```python
from build123d import *

# Parameters (mm, degrees)
CUT_EXTRUDE1_START        = -45.212
CUT_EXTRUDE1_DEPTH        = 3.302
CUT_EXTRUDE1_DEPTH_BACK   = 1.5875
SKETCH4_W                 = 30.1625
SKETCH4_H                 = 23.495
BOSS_EXTRUDE1_DEPTH       = 3.175
SKETCH5_R                 = 1.524
CUT_EXTRUDE2_DEPTH        = 8.96925
F_1_0MM_DOWEL_HOLE1_D     = 1
F_1_0MM_DOWEL_HOLE1_DEPTH = 3.175


with BuildPart() as part:
    # Sketch2 → Revolve1 (revolve)
    with BuildSketch(Plane.XY):
        Polygon((45.24375, -12.7), (50.00625, -12.7), (50.00625, 9.525), (54.76875, 9.525), (54.76875, 12.7), (50.00625, 12.7), (45.24375, 12.7), align=None)
    revolve(axis=Axis((0, 12.7, 0), (0, -1, 0)))

    # Sketch3 → Cut-Extrude1 (cut, two sides)
    with BuildSketch(Plane.XY.offset(CUT_EXTRUDE1_START)) as cut_extrude1_sk:
        with BuildLine():
            Line((-15.08125, -12.7), (15.08125, -12.7))
            Line((15.08125, -12.7), (15.08125, -5.55625))
            ThreePointArc((15.08125, -5.55625), (0, 9.525), (-15.08125, -5.55625))
            Line((-15.08125, -5.55625), (-15.08125, -12.7))
        make_face()
    extrude(amount=CUT_EXTRUDE1_DEPTH, mode=Mode.SUBTRACT)
    extrude(cut_extrude1_sk.sketch, amount=-CUT_EXTRUDE1_DEPTH_BACK, mode=Mode.SUBTRACT)

    # Sketch4 → Boss-Extrude1 (add)
    with BuildSketch(Plane.XY.offset(-46.7995)):
        with BuildLine():
            ThreePointArc((15.08125, -5.55625), (0, 9.525), (-15.08125, -5.55625))
            Line((-15.08125, -5.55625), (-15.08125, -12.7))
            Line((-15.08125, -12.7), (15.08125, -12.7))
            Line((15.08125, -12.7), (15.08125, -5.55625))
        make_face()
        with Locations((0, -24.4475)):
            Rectangle(SKETCH4_W, SKETCH4_H)
    extrude(amount=-BOSS_EXTRUDE1_DEPTH)

    # Sketch5 → Cut-Extrude2 (cut, through all)
    with BuildSketch(Plane.XY.offset(-46.7995)):
        with Locations((0, -19.0881)):
            Circle(SKETCH5_R)
        with Locations((0, -9.3091)):
            Circle(SKETCH5_R)
        with BuildLine():
            Line((-3.175, -36.195), (-3.175, -28.9687))
            ThreePointArc((-3.175, -28.9687), (0, -25.7937), (3.175, -28.9687))
            Line((3.175, -28.9687), (3.175, -36.195))
            Line((3.175, -36.195), (-3.175, -36.195))
        make_face()
    extrude(amount=-CUT_EXTRUDE2_DEPTH, mode=Mode.SUBTRACT)

    # Ø1.0mm Dowel Hole1
    with Locations(Plane(origin=(0, 9.525, 0), x_dir=(-1, 0, 0), z_dir=(0, -1, 0))):
        with Locations((-35.279486504, -38.727354522), (-37.043556499, 37.043556499), (37.043556499, 37.043556499), (37.043556499, -37.043556499)):
            Hole(F_1_0MM_DOWEL_HOLE1_D / 2, depth=F_1_0MM_DOWEL_HOLE1_DEPTH)


solid = part.part
```
The model under review builds one solid part; all positions refer to its coordinate system, in mm. A direction names the side the tool comes from. Round coordinates to 2 decimals unless told otherwise and drop trailing zeros. Order: outer loops, then holes, each group sorted by start corner. A loop starts at its lowest first (then second) coordinate and runs counter-clockwise, first axis right, second up.
Item 1: Draft analysis for pull direction X (two halves, no side actions). For faces 5 (the flat face through (9, -36.195, -48)), 6 (the cylindrical face through (-7.13, 11.135, 54.303)), 7 (the flat face through (15.081, -9, -45)), 8 (the cylindrical face through (0.33, 9.52, -45.68)), state which applies: released by +X, released by -X, zero draft, split by the parting line, or undercut.
Working result:
face 5: zero draft
face 6: split by the parting line
face 7: undercut
face 8: undercut
Item 2: Machinability: for faces 1 (the flat face through (0, -13, -46.8)), 2 (the cylindrical face through (13.93, 0.22, -49.07)), 3 (the flat face through (15.081, -21, -48)), 4 (the cylindrical face through (-13.81, 0.505, -49.065)), which of the approach directions +Z, -Z, +X, -X, +Y, -Y give a long, thin tool a straight path to every point of the face, cutting with its end or side? Answer none if there is none.
Working result:
face 1: -Y
face 2: -Z, +X
face 3: -Z, +X, -Y
face 4: -Z, -X
Item 3: Add section D-D, the plane y = -2.5. State the section outline as (x, z) points, and give its area (3 significant figures).
Working result:
outline: (-14.77, -49.97) - (-1.78, -49.97) arc R50.01 ccw to (1.78, -49.97) - (14.77, -49.97) - (14.77, -47.78) arc R50.01 ccw (long way) to (-14.77, -47.78) - close; hole (-14.77, -46.8) - (14.77, -46.8) - (14.77, -42.77) arc R45.24 ccw (long way) to (-14.77, -42.77) - close
area: 1,380 mm2
Item 4: Add section A-A, the plane x = 0. Count the separate pieces of the cut face and the enclosed holes in it, and give its area (3 significant figures).
Working result:
separate pieces: 4
enclosed holes: 0
area: 260 mm2
Item 5: For pin 1 (3.5 mm diameter, centred on y = -33.5, z = -48, fed in from +X); pin 2 (3.5 mm diameter, centred on y = -33, z = -48.5, fed in from -X); pin 3 (3.5 mm diameter, centred on y = -8.5, z = -44, fed in from +X), all flat-tipped, find the tip position at first contact; note any pin that passes through.
Working result:
pin 1: stops at x = 15.08
pin 2: stops at x = -15.08
pin 3: stops at x = 26.75
Item 6: To check wall thickness, follow probe 1 along Y at (x, z) = (38, 25.5); probe 2 along Y at (x, z) = (-30, 42.5) (3 decimals); probe 3 along Z at (x, y) = (-26.5, 9). State the ranges of each line that lie inside material, in increasing order.
Working result:
probe 1: y = -12.7 to 12.7
probe 2: y = 9.525 to 12.7
probe 3: z = -42.41 to -36.67, 36.67 to 42.41
Item 7: Add section C-C, the plane x = 32. State the section outline as (y, z) points (3 decimals), and give its area (3 significant figures).
Working result:
outline: (-12.7, -38.427) - (9.525, -38.427) - (9.525, -44.448) - (12.7, -44.448) - (12.7, -31.984) - (-12.7, -31.984) - close; (-12.7, 31.984) - (12.7, 31.984) - (12.7, 44.448) - (9.525, 44.448) - (9.525, 38.427) - (-12.7, 38.427) - close
area: 366 mm2
Item 8: Add section B-B, the plane z = 41. State the section outline as (x, y) points (3 decimals).
Working result:
outline: (-36.313, 9.525) - (-28.629, 9.525) - (-28.629, -12.7) - (-19.131, -12.7) - (-19.131, 12.7) - (-36.313, 12.7) - close; (19.131, -12.7) - (28.629, -12.7) - (28.629, 9.525) - (36.313, 9.525) - (36.313, 12.7) - (19.131, 12.7) - close
